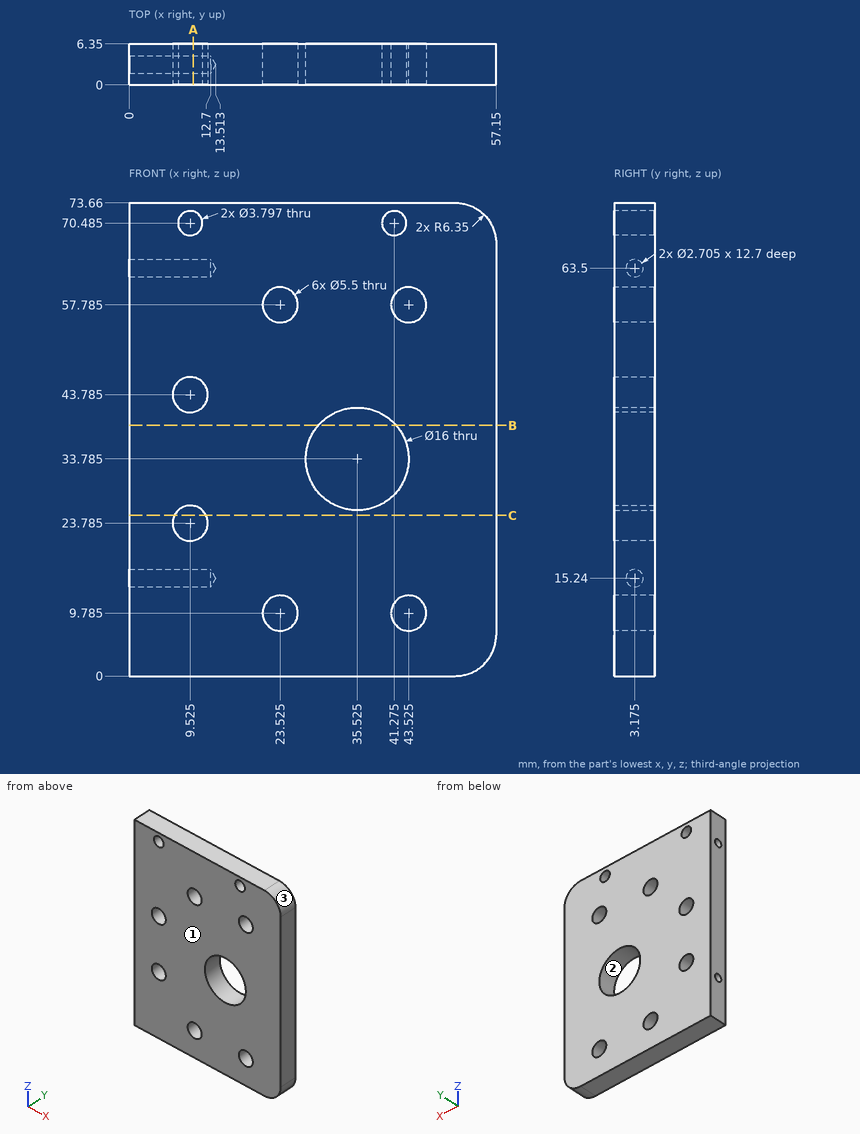
The drawing under review shows one solid part. Ordinate dimensions are in mm from its lowest x, y, z. Coordinates: 2 decimals unless noted, no trailing zeros. Write each loop counter-clockwise with the first axis right and the second up, starting at its lowest first coordinate (ties: lowest second). Pieces come first, ordered by that corner, then holes. Notation, with made-up numbers: (87.5, 36.5) - (99.5, 36.5) arc R14 ccw to (99.5, 62.5) - close; hole circle Ø11 at (16, -0.75). An arc over 180 degrees is marked (long way). Answer as CSV lines item,"result".
(1) We need section C-C (z = 25). Give the boundary of the cut face in (x, y).
Data:
outline,"(0, 0) - (7.06, 0) - (7.06, 6.35) - (0, 6.35) - close; (11.99, 0) - (57.15, 0) - (57.15, 6.35) - (11.99, 6.35) - close"
(2) Mouldability with a two-part tool opening along X and no side actions: class the marked faces 1, 2 and 3 as pulls with the +X half, pulls with the -X half, needs draft (parallel to the pull), parting line crosses it, or undercut.
Data:
face 1,"needs draft"
face 2,"undercut"
face 3,"pulls with the +X half"
(3) We need section A-A (x = 10). Count the separate pieces of the cut face and the enclosed holes in it, plus the area to 3 significant figures.
Data:
separate pieces,"4"
enclosed holes,"2"
area,"364 mm2"
(4) For line 1 along Z through (x, y) = (9.5, 5.5) (1 decimal); line 2 along X through (y, z) = (5, 8); line 3 along Z through (x, y) = (26, 2.75) (1 decimal), list the stretches that pass through material, from the lowest coordinate up. Write a range as [from, to].
Data:
line 1,"z = [0, 21], [26.5, 41], [46.5, 68.6], [72.4, 73.7]"
line 2,"x = [0, 21.43], [25.62, 41.43], [45.62, 57.15]"
line 3,"z = [0, 8.6], [11, 56.6], [59, 73.7]"
(5) Clearance check with flat-ended pins moving along their axes: pin 1 Ø18.5 at (x, z) = (35.525, 33.785) entering from +Y; pin 2 Ø2 at (y, z) = (3.175, 15.24) entering from -X. State where each tip first meets the part, or that it passes through.
Data:
pin 1,"stops at y = 6.35"
pin 2,"stops at x = 12.91"
(6) We need section B-B (z = 39). Give the boundary of the cut face in (x, y).
Data:
outline,"(0, 0) - (29.46, 0) - (29.46, 6.35) - (0, 6.35) - close; (41.59, 0) - (57.15, 0) - (57.15, 6.35) - (41.59, 6.35) - close"
